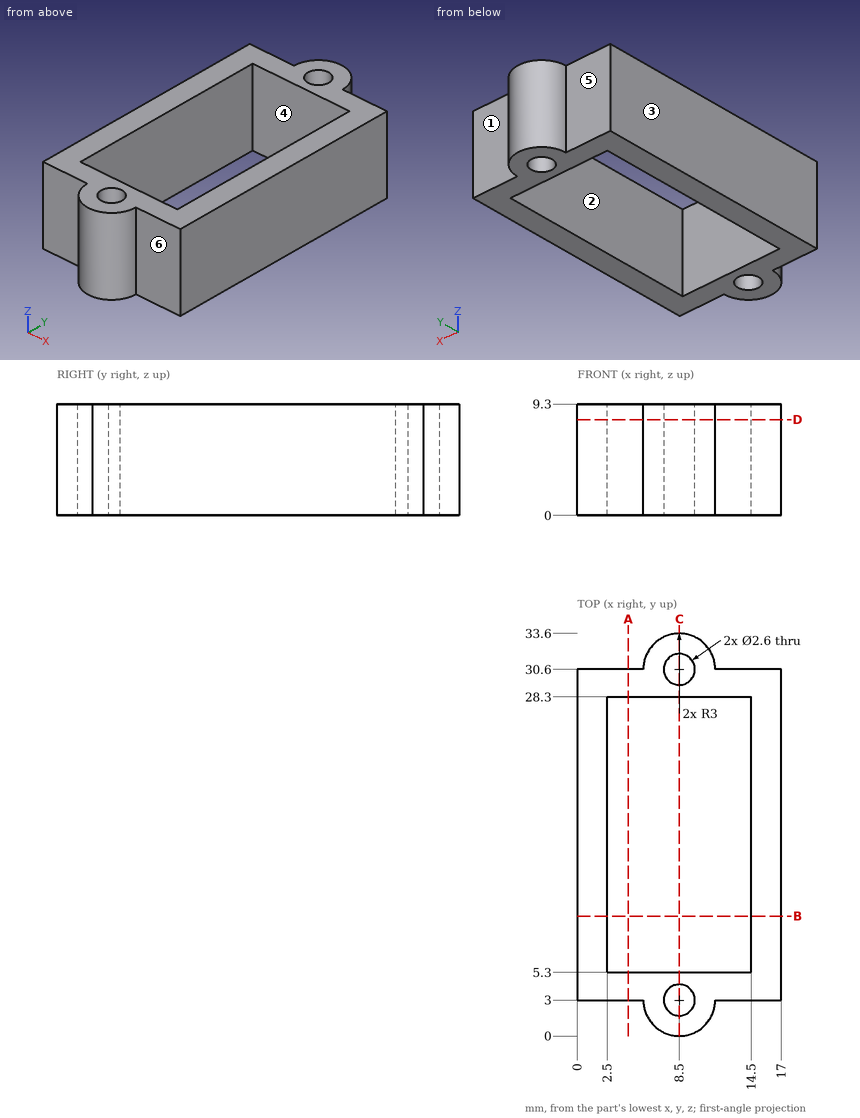
Job drawing, mm, ordinate dimensions from the low corner. One solid piece. A direction names the side the tool comes from. Coordinates: 2 decimals unless noted, no trailing zeros. Order: outer loops, then holes, each group sorted by start corner. A loop starts at its lowest first (then second) coordinate and runs counter-clockwise, first axis right, second up. Notation, with made-up numbers: (9, 56.25) -> (49, 56.25) arc R29 ccw to (49, 89.25) -> close; hole circle Ø9 at (17.25, 3). An arc over 180 degrees is marked (long way). Return JSON: item names as keys, results as strings. Group by question number.
Item 1: Saw through at B-B on y = 10. Write the cut outline in (x, z), then the cut area to 3 significant figures.
Item 2: Pull direction X, two halves, no side cores. Call the marked faces 1, 2 and 3: pulls with the +X half, pulls with the -X half, needs draft (parallel to the pull), parting line crosses it, or undercut.
Item 3: Saw through at C-C on x = 8.5. Write the cut outline in (y, z), then the cut area to 3 significant figures.
Item 4: Saw through at A-A on x = 4.25. Write the cut outline in (y, z), then the cut area to 3 significant figures.
Item 5: Wall check: line 1 along Y through (x, z) = (8.5, 6); line 2 along X through (y, z) = (14.5, 2.75); line 3 along Y through (x, z) = (15.5, 8). Give the ranges that are in metal, low to high. Write a range as [from, to].
Item 6: Flat gauge pins, fed straight in: P1, Ø3, axis at x = 8.5, y = 3, coming from the +Z side; P2, Ø1.6, axis at x = 3, z = 5, coming from the +Y side; P3, Ø3, axis at x = 13.5, z = 3.5, coming from the -Y side. Where does each tip first touch, or does it go through?
Item 7: Tool access for the marked faces 4, 5 and 6: list every direction of +Z, -Z, +X, -X, +Y, -Y with a clear straight run to the whole face (end or side of a thin tool).
Item 8: Saw through at D-D on z = 8. Write the cut outline in (x, y), then the cut area to 3 significant figures.
Values found:
{
 "1": {"outline": "(0, 0) -> (2.5, 0) -> (2.5, 9.3) -> (0, 9.3) -> close; (14.5, 0) -> (17, 0) -> (17, 9.3) -> (14.5, 9.3) -> close", "area": "46.5 mm2"},
 "2": {"face 1": "needs draft", "face 2": "undercut", "face 3": "pulls with the -X half"},
 "3": {"outline": "(0, 0) -> (1.7, 0) -> (1.7, 9.3) -> (0, 9.3) -> close; (4.3, 0) -> (5.3, 0) -> (5.3, 9.3) -> (4.3, 9.3) -> close; (28.3, 0) -> (29.3, 0) -> (29.3, 9.3) -> (28.3, 9.3) -> close; (31.9, 0) -> (33.6, 0) -> (33.6, 9.3) -> (31.9, 9.3) -> close", "area": "50.2 mm2"},
 "4": {"outline": "(3, 0) -> (5.3, 0) -> (5.3, 9.3) -> (3, 9.3) -> close; (28.3, 0) -> (30.6, 0) -> (30.6, 9.3) -> (28.3, 9.3) -> close", "area": "42.8 mm2"},
 "5": {"line 1": "y = [0, 1.7], [4.3, 5.3], [28.3, 29.3], [31.9, 33.6]", "line 2": "x = [0, 2.5], [14.5, 17]", "line 3": "y = [3, 30.6]"},
 "6": {"P1": "stops at z = 9.3", "P2": "stops at y = 30.6", "P3": "stops at y = 3"},
 "7": {"face 4": "+Z, -Z", "face 5": "+Z, -Z, -X, +Y", "face 6": "+Z, -Z, +X, -Y"},
 "8": {"outline": "(0, 3) -> (5.5, 3) arc R3 ccw to (11.5, 3) -> (17, 3) -> (17, 30.6) -> (11.5, 30.6) arc R3 ccw to (5.5, 30.6) -> (0, 30.6) -> close; hole (2.5, 5.3) -> (14.5, 5.3) -> (14.5, 28.3) -> (2.5, 28.3) -> close; hole circle Ø2.6 at (8.5, 3); hole circle Ø2.6 at (8.5, 30.6)", "area": "211 mm2"}
}
